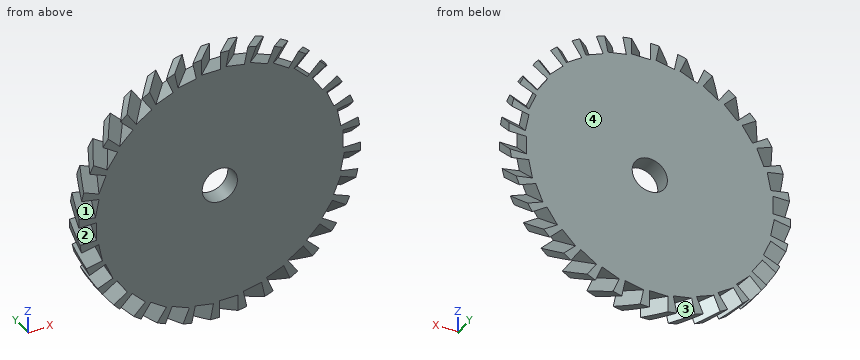
from build123d import *

# Parameters (mm, degrees)
SKETCH1_R           = 50.8
SKETCH1_R_2         = 6.35
BOSS_EXTRUDE1_DEPTH = 6.35
CUT_EXTRUDE1_DEPTH  = 6.35
CIRPATTERN1_COUNT   = 32


with BuildPart() as part:
    # Sketch1 → Boss-Extrude1 (new body)
    with BuildSketch(Plane(origin=(0, 0, 0), x_dir=(1, 0, 0), z_dir=(0, 1, 0))):
        with Locations(Location((0, 0, 0), (0, 0, 270))):
            Circle(SKETCH1_R)
        with Locations(Location((0, 0, 0), (0, 0, 270))):
            Circle(SKETCH1_R_2, mode=Mode.SUBTRACT)
    extrude(amount=BOSS_EXTRUDE1_DEPTH)

    # Sketch2 → Cut-Extrude1 (cut)
    with BuildSketch(Plane.XY.offset(50.8)):
        Polygon((15.154182204, 14.961586159), (-11.786586159, -11.979182204), (-15.154182204, -8.611586159), (11.786586159, 18.329182204), align=None)
    cut_extrude1 = extrude(amount=-CUT_EXTRUDE1_DEPTH, mode=Mode.SUBTRACT)

    # CirPattern1: Cut-Extrude1 ×32 about axis
    cirpattern1_axis = Axis((0, 0, 0), (0, 1, 0))
    for i in range(1, CIRPATTERN1_COUNT):
        add(cut_extrude1.rotate(cirpattern1_axis, i * 360 / CIRPATTERN1_COUNT), mode=Mode.SUBTRACT)


solid = part.part
Could you check a few things on this model? Use its own coordinates, in mm. Face numbers are marked on the shaded views. A direction names the side the tool comes from. Round coordinates to 2 decimals unless told otherwise and drop trailing zeros. Write each loop counter-clockwise with the first axis right and the second up, starting at its lowest first coordinate (ties: lowest second). Pieces come first, ordered by that corner, then holes. Notation, with made-up numbers: (45.5, 24.5) - (83.5, 24.5) arc R32 ccw to (83.5, 52.5) - close; hole circle Ø11 at (7.5, -4). An arc over 180 degrees is marked (long way). Put each result on its own line as item: value. Start each with the question number.
(1) I want a section at A-A, the plane z = 21. Please give me the cut outline in (x, y).
(2) For the marked faces 3 and 4, which set-ups out of +Z, -Z, +X, -X, +Y, -Y let a thin tool reach every point of the face, with its end or its side?
(3) Thinking about a two-plate mould opening in X: for the marked faces 1 and 2, which applies, released by +X, released by -X, zero draft, split by the parting line, or undercut?
(4) Will these pins go through, and if not, where does the flat tip stop? pin 1 (1.9 mm diameter, centred on y = 2, z = -2.5, fed in from -X); pin 2 (3 mm diameter, centred on x = -33, y = 2, fed in from +Z).
(5) I need wall thicknesses on probe 1 along X at (y, z) = (5.25, 0); probe 2 along X at (y, z) = (3.25, -30.5); probe 3 along X at (y, z) = (2.5, 37). Which ranges of each line are inside material? Lowest first, please.
Here are the results:
1. outline: (-46.26, 0) - (-43.21, 0) - (-39.43, 2.1) - (-39.43, 0) - (39.41, 0) - (39.41, 2.22) - (46.26, 4.84) - (46.26, 6.35) - (43.21, 6.35) - (39.43, 4.25) - (39.43, 6.35) - (-39.41, 6.35) - (-39.41, 4.13) - (-46.26, 1.51) - close
2. face 3: -Z, +Y
2. face 4: +Z, -Z, +X, -X, +Y
3. face 1: undercut
3. face 2: zero draft
4. pin 1: stops at x = -44.45
4. pin 2: stops at z = 39.81
5. probe 1: x = -44.45 to -6.35, 6.35 to 44.45
5. probe 2: x = -39.72 to -35.37, -32.36 to 32.36, 35.16 to 39.45
5. probe 3: x = -33.19 to -29.58, -24.63 to 24.63, 27.96 to 31.28
